```python
from build123d import *

# Parameters (mm, degrees)
F0_R      = 39.988353
F1_DEPTH  = 25.4
F1_FACE_R = 39.988353
F2_DEPTH  = 50.8
F3_R      = 20.704391
F4_DEPTH  = 76.201
F5_W      = 66.406839
F5_H      = 39.493055
F6_DEPTH  = 25.4


with BuildPart() as f1:
    # F0 (on Front) → F1 (new body)
    with BuildSketch(Plane.XZ):
        with Locations((40.370677, 4.534387)):
            Circle(F0_R)
    extrude(amount=F1_DEPTH)

    # F1_face (on face) → F2 (join)
    with BuildSketch(Plane(origin=(40.370677, -25.4, 4.534387), x_dir=(1, 0, 0), z_dir=(0, -1, 0))):
        Circle(F1_FACE_R)
    extrude(amount=F2_DEPTH)

    # F3 (on face) → F4 (cut, through all)
    with BuildSketch(Plane.XZ.offset(76.2)):
        with Locations((39.785597, 4.241847)):
            Circle(F3_R)
    extrude(amount=-F4_DEPTH, mode=Mode.SUBTRACT)

    # F5 (on Front) → F6 (join)
    with BuildSketch(Plane.XZ):
        with Locations((-22.640213, 0.292541)):
            Rectangle(F5_W, F5_H)
    extrude(amount=F6_DEPTH)


solid = f1.part
```
Input: part model. Units: mm. Frame: model coordinates. A direction names the side the tool comes from. Round coordinates to 2 decimals unless told otherwise and drop trailing zeros. Order: outer loops, then holes, each group sorted by start corner. A loop starts at its lowest first (then second) coordinate and runs counter-clockwise, first axis right, second up. Notation, with made-up numbers: (-10.5, 41) - (6.5, 41) arc R11 cw to (6.5, 57) - close; hole circle Ø9 at (-36.75, 4.5). An arc over 180 degrees is marked (long way). One line per question, with ' | ' between items. Start each with the question number.
1) Set-up query: faces 1 (the flat face through (58, -76.2, -13)), 2 (the flat face through (-24, -13, -19.454)). Return all of +Z, -Z, +X, -X, +Y, -Y with unobstructed straight access to the full face (end or side cutting, diameter ignored); none if empty.
2) Cut plane D-D, the plane y = -18. Return the cut outline in (x, z), then the cut area to 3 significant figures.
3) Cut plane A-A, the plane x = 28. Return the cut outline in (y, z), then the cut area to 3 significant figures.
4) Contact query for flat-ended pins moving along their axis: P1, Ø6, axis at x = 14.5, y = -61.5, coming from the +Z side; P2, Ø20.5, axis at x = -26, y = -13.5, coming from the -Z side; P3, Ø2, axis at x = -14.5, y = -13, coming from the +Z side; P4, Ø10, axis at x = 26.5, z = 7.5, coming from the -Y side. Output: stop coordinate, or through.
5) Cut plane C-C, the plane x = -30.5. Return the cut outline in (y, z).
6) Ray query, probe 1 along Y at (x, z) = (-18, -17.5); probe 2 along Z at (x, y) = (-47.5, -10.5); probe 3 along Z at (x, y) = (44.5, -15). Return the intervals inside material, ascending.
7) Pull-direction query (Z, two-part tool) for faces 3 (the flat face through (-27, -13, 20.039)), 4 (the cylindrical face through (58.91, -38.63, -3.69)), 5 (the flat face through (-55.844, -13, 0)); classes: +Z half, -Z half, draft (parallel to the pull), parting line (faces both ways), or undercut.
8) Cut plane B-B, the plane z = 18. Return the cut outline in (x, y), then the cut area to 3 significant figures.
Worked out:
1) face 1: +Z, -Z, +X, -X, -Y | face 2: -Z, -X, +Y, -Y
2) outline: (-55.84, -19.45) - (8.38, -19.45) arc R39.99 ccw (long way) to (3.51, 20.04) - (-55.84, 20.04) - close; hole circle Ø41.41 at (39.79, 4.24) | area: 5,970 mm^2
3) outline: (-76.2, -33.49) - (0, -33.49) - (0, -12.78) - (-76.2, -12.78) - close; (-76.2, 21.26) - (0, 21.26) - (0, 42.56) - (-76.2, 42.56) - close | area: 3,200 mm^2
4) P1: stops at z = 37.34 | P2: stops at z = -19.45 | P3: stops at z = 20.04 | P4: passes through
5) outline: (-25.4, -19.45) - (0, -19.45) - (0, 20.04) - (-25.4, 20.04) - close
6) probe 1: y = -25.4 to 0 | probe 2: z = -19.45 to 20.04 | probe 3: z = -35.24 to -15.92, 24.4 to 44.31
7) face 3: +Z half | face 4: undercut | face 5: draft
8) outline: (-55.84, -25.4) - (2.72, -25.4) - (2.72, -76.2) - (24.31, -76.2) - (24.31, 0) - (-55.84, 0) - close; (55.26, -76.2) - (78.02, -76.2) - (78.02, 0) - (55.26, 0) - close | area: 4,870 mm^2
